CAD build for the part. Positions are in the model's coordinates, mm. Face numbers are marked on the shaded views. Give positions to 0.01 mm unless a question says otherwise; leave off trailing zeros. Order: outer loops, then holes, each group sorted by start corner. A loop starts at its lowest first (then second) coordinate and runs counter-clockwise, first axis right, second up.
```python
from build123d import *

# Parameters (mm, degrees)
SKETCH1_W           = 16
SKETCH1_H           = 80
SKETCH1_R           = 4
SKETCH1_R_2         = 1.625
BOSS_EXTRUDE1_DEPTH = 5
FILLET1_R           = 2


with BuildPart() as part:
    # Sketch1 → Boss-Extrude1 (new body)
    with BuildSketch(Plane.XY):
        with Locations((8, 40)):
            Rectangle(SKETCH1_W, SKETCH1_H)
        with Locations((8, 72)):
            Circle(SKETCH1_R, mode=Mode.SUBTRACT)
        with Locations((8, 8)):
            Circle(SKETCH1_R, mode=Mode.SUBTRACT)
        with Locations((8, 20)):
            Circle(SKETCH1_R_2, mode=Mode.SUBTRACT)
        with Locations((8, 60)):
            Circle(SKETCH1_R_2, mode=Mode.SUBTRACT)
        with BuildLine():
            Line((6.5, 50.5), (9.5, 50.5))
            ThreePointArc((9.5, 50.5), (10.75, 49.25), (9.5, 48))
            Line((9.5, 48), (6.5, 48))
            ThreePointArc((6.5, 48), (5.25, 49.25), (6.5, 50.5))
        make_face(mode=Mode.SUBTRACT)
        with BuildLine():
            Line((6.5, 43), (9.5, 43))
            ThreePointArc((9.5, 43), (10.75, 41.75), (9.5, 40.5))
            Line((9.5, 40.5), (6.5, 40.5))
            ThreePointArc((6.5, 40.5), (5.25, 41.75), (6.5, 43))
        make_face(mode=Mode.SUBTRACT)
    extrude(amount=BOSS_EXTRUDE1_DEPTH)

    # Fillet1
    fillet1_edges = [part.edges().sort_by_distance(p)[0] for p in [
        (0, 80, 2.5),
        (16, 80, 2.5),
        (16, 0, 2.5),
        (0, 0, 2.5),
    ]]
    fillet(fillet1_edges, radius=FILLET1_R)


solid = part.part
```
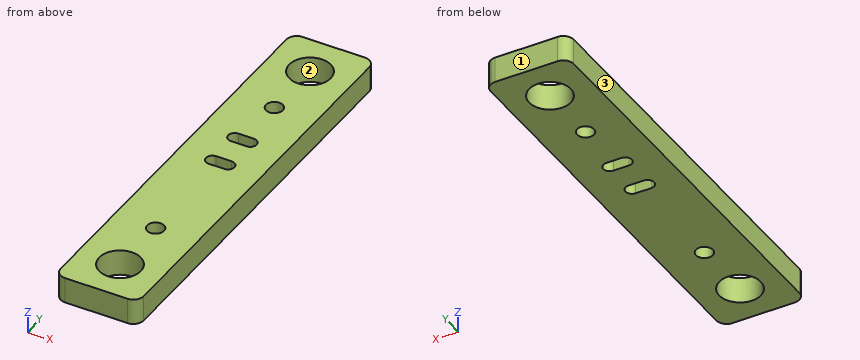
Item 1: Wall check: L1, parallel to Y at x = 6, z = 4.35; L2, parallel to Y at x = 10.25, z = 0.6; L3, parallel to X at y = 5, z = 2.45. Give the ranges that are in metal, low to high.
Item 2: Drop a flat-ended pin along its axis: pin 1 Ø7 at (x, y) = (8, 8) entering from +Z. Give the stop position or say it passes through.
Item 3: Slice it at A-A (y = 60). Give the cut face in (x, z) (3 decimals).
Item 4: Slice it at D-D (y = 72). Give the cut face in (x, z).
Item 5: Two-plate mould, pull along X, no slides. Class the marked faces 1, 2 and 3: released by +X, released by -X, zero draft, split by the parting line, or undercut.
Item 6: Slice it at C-C (x = 8). Give the cut face in (y, z) (3 decimals), and give its area (4 significant figures).
Item 7: Slice it at B-B (z = 3.55). Give the cut face in (x, y) (3 decimals), and give its area (3 significant figures).
A:
1. L1: y = 0 to 4.54, 11.46 to 40.6, 42.9 to 48.1, 50.4 to 68.54, 75.46 to 80
1. L2: y = 0 to 4.69, 11.31 to 40.75, 42.75 to 48.25, 50.25 to 68.69, 75.31 to 80
1. L3: x = 0 to 5.35, 10.65 to 16
2. pin 1: passes through
3. outline: (0, 0) - (6.375, 0) - (6.375, 5) - (0, 5) - close; (9.625, 0) - (16, 0) - (16, 5) - (9.625, 5) - close
4. outline: (0, 0) - (4, 0) - (4, 5) - (0, 5) - close; (12, 0) - (16, 0) - (16, 5) - (12, 5) - close
5. face 1: zero draft
5. face 2: undercut
5. face 3: released by -X
6. outline: (0, 0) - (4, 0) - (4, 5) - (0, 5) - close; (12, 0) - (18.375, 0) - (18.375, 5) - (12, 5) - close; (21.625, 0) - (40.5, 0) - (40.5, 5) - (21.625, 5) - close; (43, 0) - (48, 0) - (48, 5) - (43, 5) - close; (50.5, 0) - (58.375, 0) - (58.375, 5) - (50.5, 5) - close; (61.625, 0) - (68, 0) - (68, 5) - (61.625, 5) - close; (76, 0) - (80, 0) - (80, 5) - (76, 5) - close
6. area: 262.5 mm2
7. outline: (0, 2) arc R2 ccw to (2, 0) - (14, 0) arc R2 ccw to (16, 2) - (16, 78) arc R2 ccw to (14, 80) - (2, 80) arc R2 ccw to (0, 78) - close; hole circle Ø8 at (8, 8); hole circle Ø8 at (8, 72); hole circle Ø3.25 at (8, 20); hole circle Ø3.25 at (8, 60); hole (6.5, 40.5) - (9.5, 40.5) arc R1.25 ccw to (9.5, 43) - (6.5, 43) arc R1.25 ccw to start; hole (6.5, 48) - (9.5, 48) arc R1.25 ccw to (9.5, 50.5) - (6.5, 50.5) arc R1.25 ccw to start
7. area: 1,130 mm2
